Work out the finished part from the listing and answer in its coordinate system (mm). A direction names the side the tool comes from. Round coordinates to 2 decimals unless told otherwise and drop trailing zeros. Write each loop counter-clockwise with the first axis right and the second up, starting at its lowest first coordinate (ties: lowest second). Pieces come first, ordered by that corner, then holes. Notation, with made-up numbers: (5.5, 17) - (39.5, 17) arc R14 ccw to (39.5, 40) - close; hole circle Ø10 at (41, 31). An arc over 180 degrees is marked (long way). Answer as a JSON object with one key per item and string values.
```python
from build123d import *

# Parameters (mm, degrees)
SKETCH1_R           = 2.6
BOSS_EXTRUDE1_DEPTH = 22
SKETCH2_W           = 200
SKETCH2_H           = 80
BOSS_EXTRUDE2_DEPTH = 4
SKETCH3_W           = 8
SKETCH3_H           = 35
CUT_EXTRUDE1_DEPTH  = 209.42744541
CHAMFER1_SIZE       = 0.5
BOSS_EXTRUDE3_START = -22
SKETCH4_W           = 8
SKETCH4_H           = 20
SKETCH4_R           = 2
BOSS_EXTRUDE3_DEPTH = 10
SKETCH5_W           = 56
SKETCH5_H           = 55
CUT_EXTRUDE2_DEPTH  = 7
FILLET1_R           = 2
SKETCH7_W           = 76
SKETCH7_H           = 8
SKETCH7_R           = 1.5
BOSS_EXTRUDE4_DEPTH = 10


with BuildPart() as part:
    # Sketch1 → Boss-Extrude1 (new body)
    with BuildSketch(Plane.XY):
        with BuildLine():
            Line((-6.63831163, 6.934898608), (-40, -25))
            Line((-40, -25), (40, -25))
            Line((40, -25), (6.63831163, 6.934898608))
            ThreePointArc((6.63831163, 6.934898608), (0, 9.6), (-6.63831163, 6.934898608))
        make_face()
        Circle(SKETCH1_R, mode=Mode.SUBTRACT)
    extrude(amount=BOSS_EXTRUDE1_DEPTH)

    # Sketch2 → Boss-Extrude2 (add)
    with BuildSketch(Plane(origin=(0, -25, 0), x_dir=(-1, 0, 0), z_dir=(0, -1, 0))):
        with Locations((0, -11)):
            Rectangle(SKETCH2_W, SKETCH2_H)
    extrude(amount=BOSS_EXTRUDE2_DEPTH)

    # Sketch3 → Cut-Extrude1 (cut, through all)
    with BuildSketch(Plane(origin=(100, 0, 0), x_dir=(0, 0, -1), z_dir=(1, 0, 0))):
        with Locations((-11, -7.5)):
            Rectangle(SKETCH3_W, SKETCH3_H)
    extrude(amount=-CUT_EXTRUDE1_DEPTH, mode=Mode.SUBTRACT)

    # Chamfer1
    chamfer1_edges = [part.edges().sort_by_distance(p)[0] for p in [
        (-2.6, 0, 0),
        (-2.6, 0, 22),
    ]]
    chamfer(chamfer1_edges, length=CHAMFER1_SIZE)

    # Sketch4 → Boss-Extrude3 (add)
    # profile 1 of 2: a face of its own
    with BuildSketch(Plane(origin=(0, 0, -29), x_dir=(-1, 0, 0), z_dir=(0, 0, -1)).offset(BOSS_EXTRUDE3_START)):
        with Locations((96, -15)):
            Rectangle(SKETCH4_W, SKETCH4_H)
        with Locations((96.4, -20)):
            Circle(SKETCH4_R, mode=Mode.SUBTRACT)
        with Locations((96.4, -10.2)):
            Circle(SKETCH4_R, mode=Mode.SUBTRACT)
    # profile 2 of 2: a face of its own
    with BuildSketch(Plane(origin=(0, 0, -29), x_dir=(-1, 0, 0), z_dir=(0, 0, -1)).offset(BOSS_EXTRUDE3_START)):
        with Locations((48, -15)):
            Rectangle(SKETCH4_W, SKETCH4_H)
        with Locations(Location((47.6, -20, 0), (0, 0, 180))):
            Circle(SKETCH4_R, mode=Mode.SUBTRACT)
        with Locations(Location((47.6, -10.2, 0), (0, 0, 180))):
            Circle(SKETCH4_R, mode=Mode.SUBTRACT)
    extrude(amount=BOSS_EXTRUDE3_DEPTH)

    # Sketch5 → Cut-Extrude2 (cut)
    with BuildSketch(Plane(origin=(0, -25, 0), x_dir=(1, 0, 0), z_dir=(0, 1, 0))):
        with Locations((-72, -23.5)):
            Rectangle(SKETCH5_W, SKETCH5_H)
    extrude(amount=-CUT_EXTRUDE2_DEPTH, mode=Mode.SUBTRACT)

    # Fillet1
    fillet1_edges = [part.edges().sort_by_distance(p)[0] for p in [
        (-100, -5, -12),
        (-92, -5, -12),
        (-44, -5, -12),
        (-52, -5, -12),
        (-44, -25, -12),
        (0, -25, 0),
        (0, -25, 15),
        (-40, -25, 18.5),
        (0, -25, 7),
        (-40, -25, 3.5),
        (0, -25, 22),
        (40, -25, 3.5),
        (40, -25, 18.5),
        (100, -27, -29),
        (100, -27, 51),
        (-100, -27, -29),
        (-44, -27, -4),
        (-44, -27, 51),
        (-100, -27, -4),
    ]]
    fillet(fillet1_edges, radius=FILLET1_R)

    # Sketch7 → Boss-Extrude4 (add)
    with BuildSketch(Plane(origin=(100, 0, 0), x_dir=(0, 0, -1), z_dir=(1, 0, 0))):
        with Locations((-11, -21)):
            Rectangle(SKETCH7_W, SKETCH7_H)
        with Locations((-41.4, -21)):
            Circle(SKETCH7_R, mode=Mode.SUBTRACT)
        with Locations((-26.2, -21)):
            Circle(SKETCH7_R, mode=Mode.SUBTRACT)
        with Locations((-11, -21)):
            Circle(SKETCH7_R, mode=Mode.SUBTRACT)
        with Locations((4.2, -21)):
            Circle(SKETCH7_R, mode=Mode.SUBTRACT)
        with Locations((19.4, -21)):
            Circle(SKETCH7_R, mode=Mode.SUBTRACT)
    extrude(amount=-BOSS_EXTRUDE4_DEPTH)


solid = part.part
```
Item 1: For faces 1 (the flat face through (95, -21, -27)), 2 (the flat face through (95, -17, 12)), 3 (the flat face through (-1, -10, 22)), 4 (the flat face through (90, -23, 12)), 5 (the flat face through (1, -11, 15)), determine the directions among +Z, -Z, +X, -X, +Y, -Y from which every point of the face is accessible in a straight line to the end or side of a thin tool.
Results found:
{"face 1": "-Z, +X, -X, +Y", "face 2": "+Z, -Z, +X, +Y", "face 3": "+Z, -X, +Y", "face 4": "+Z, -Z, +Y", "face 5": "-X, +Y"}
Item 2: Determine the mould class of faces 6 (the flat face through (-22.8, -8.535, 3.442)), 7 (the flat face through (-96, -15, -7)), 8 (the cylindrical face through (-0.338, 2.578, 18.204)), 9 (the cylindrical face through (-49.598, -20.088, -11.93)) for opening direction Y: pulls with the +Y half, pulls with the -Y half, needs draft (parallel to the pull), parting line crosses it, or undercut.
Results found:
{"face 6": "pulls with the +Y half", "face 7": "needs draft", "face 8": "undercut", "face 9": "undercut"}
Item 3: A cutting plane is placed at C-C (y = 0). Write down the section's boundary in (x, z).
Results found:
{"outline": "(-13.88, 0) - (-3.1, 0) - (-2.6, 0.5) - (-2.6, 7) - (-13.88, 7) - close; (-13.88, 15) - (-2.6, 15) - (-2.6, 21.5) - (-3.1, 22) - (-13.88, 22) - close; (2.6, 0.5) - (3.1, 0) - (13.88, 0) - (13.88, 7) - (2.6, 7) - close; (2.6, 15) - (13.88, 15) - (13.88, 22) - (3.1, 22) - (2.6, 21.5) - close"}
Item 4: A cutting plane is placed at B-B (z = 31.5). Write down the section's boundary in (x, y).
Results found:
{"outline": "(-44, -29) - (100, -29) - (100, -17) - (90, -17) - (90, -25) - (-44, -25) - close"}
Item 5: A cutting plane is placed at A-A (x = 0). Write down the section's boundary in (y, z), and give its area (3 significant figures).
Results found:
{"outline": "(-29, -29) - (-25, -29) - (-25, -2) arc R2 cw to (-23, 0) - (-3.1, 0) - (-2.6, 0.5) - (-2.6, 7) - (-23, 7) arc R2 cw to (-25, 9) - (-25, 13) arc R2 cw to (-23, 15) - (-2.6, 15) - (-2.6, 21.5) - (-3.1, 22) - (-23, 22) arc R2 cw to (-25, 24) - (-25, 51) - (-29, 51) - close; (2.6, 0.5) - (3.1, 0) - (9.6, 0) - (9.6, 7) - (2.6, 7) - close; (2.6, 15) - (9.6, 15) - (9.6, 22) - (3.1, 22) - (2.6, 21.5) - close", "area": "735 mm²"}
Item 6: Each of these flat-tipped pins is pushed along its axis until it touches: P1, Ø1.2, axis at x = -95.5, z = -14, coming from the +Y side; P2, Ø5, axis at x = 93, z = 1.5, coming from the +Y side; P3, Ø16.5, axis at x = 13, y = -5, coming from the +Z side. Where does it stop, or does it pass through?
Results found:
{"P1": "y = -5", "P2": "y = -17", "P3": "z = 22"}
Item 7: Consider line 1 along Y through (x, z) = (-47.6, -12.5); line 2 along Y through (x, z) = (94.25, -4.2); line 3 along Z through (x, y) = (-9.5, -18.5). Determine where each line is inside the solid, lowest interval first.
Results found:
{"line 1": "-29 to -22, -18 to -12.2, -8.2 to -5", "line 2": "-29 to -22.5, -19.5 to -17", "line 3": "0 to 7, 15 to 22"}
Item 8: A cutting plane is placed at D-D (x = 34). Write down the section's boundary in (y, z).
Results found:
{"outline": "(-29, -29) - (-25, -29) - (-25, -2) arc R2 cw to (-23, 0) - (-19.26, 0) - (-19.26, 7) - (-23, 7) arc R2 cw to (-25, 9) - (-25, 13) arc R2 cw to (-23, 15) - (-19.26, 15) - (-19.26, 22) - (-23, 22) arc R2 cw to (-25, 24) - (-25, 51) - (-29, 51) - close"}
